Work out the finished part from the listing and answer in its coordinate system (mm). Face numbers are marked on the shaded views. A direction names the side the tool comes from. Coordinates: 2 decimals unless noted, no trailing zeros. Write each loop counter-clockwise with the first axis right and the second up, starting at its lowest first coordinate (ties: lowest second). Pieces come first, ordered by that corner, then holes. Notation, with made-up numbers: M -2,-2.75 L 16,-2.75 A8 ccw 16,3.25 Z; hole C 48,-17.75 d4. An arc over 180 degrees is marked long. Answer as CSV lines item,"result". Start each with the question number.
(1) A cutting plane is placed at C-C on z = -14. Give the vertices of the cut face in (x, y).
(2) A cutting plane is placed at A-A on x = 25. Give the vertices of the cut face in (y, z).
(3) For the marked faces 1 and 2, determine the directions among +Z, -Z, +X, -X, +Y, -Y from which every point of the face is accessible in a straight line to the end or side of a thin tool.
(4) Flat-ended cylindrical pins translate along their axes: P1, Ø1.4, axis at y = -2.37, z = -7.24, coming from the +X side; P2, Ø6, axis at x = 18.5, z = -132, coming from the +Y side; P3, Ø1.5, axis at x = 47.5, y = -3, coming from the +Z side; P4, Ø2, axis at y = -6.71, z = -3.6, coming from the -X side. Find the tip coordinate at first contact, or state that the pin passes through.
(5) A cutting plane is placed at B-B on y = 21. Give the vertices of the cut face in (x, z).
(6) Find the intervals of material crossed by L1, parallel to X at y = 9, z = -3.5; L2, parallel to X at y = -3.5, z = -79; L3, parallel to Y at x = 15, z = -22, in increasing order. Write a range as [from, to].
from build123d import *

# Parameters (mm, degrees)
BOSS_EXTRUDE1_DEPTH = 17.78
SKETCH2_R           = 10
CUT_EXTRUDE2_DEPTH  = 5.08
SKETCH8_R           = 0.75
SKETCH8_R_2         = 0.724827396
SKETCH8_R_3         = 0.742534986
CUT_EXTRUDE7_DEPTH  = 5.08
BOSS_EXTRUDE2_DEPTH = 35.56
SKETCH7_W           = 41.148
SKETCH7_H           = 20.066
CUT_EXTRUDE5_DEPTH  = 26.797
FILLET2_R           = 2.54
FILLET3_R           = 2.54
FILLET4_R           = 2.54
FILLET5_R           = 12.7


with BuildPart() as part:
    # Sketch1 → Boss-Extrude1 (new body)
    with BuildSketch(Plane(origin=(0, 0, 0), x_dir=(0, 0, -1), z_dir=(1, 0, 0))):
        with BuildLine():
            Line((32.896583501, -19.220426478), (153.708015153, -35.416630381))
            Line((153.708015153, -35.416630381), (158.7704814, 2.345538988))
            Line((158.7704814, 2.345538988), (32.896583501, 19.220426478))
            ThreePointArc((32.896583501, 19.220426478), (-38.1, 0), (32.896583501, -19.220426478))
        make_face()
    extrude(amount=BOSS_EXTRUDE1_DEPTH)

    # Sketch2 → Cut-Extrude2 (cut)
    with BuildSketch(Plane(origin=(17.78, 0, 0), x_dir=(0, 0, -1), z_dir=(1, 0, 0))):
        Circle(SKETCH2_R)
    extrude(amount=-CUT_EXTRUDE2_DEPTH, mode=Mode.SUBTRACT)

    # Sketch8 → Cut-Extrude7 (cut)
    with BuildSketch(Plane(origin=(12.7, 0, 0), x_dir=(0, 0, -1), z_dir=(1, 0, 0))):
        with Locations((-7.236662764, 2.372912145)):
            Circle(SKETCH8_R)
        with Locations((-6.97289018, -0.615469361)):
            Circle(SKETCH8_R)
        with Locations((-6.709117597, -3.603850867)):
            Circle(SKETCH8_R)
        with Locations((-2.372912145, -7.236662764)):
            Circle(SKETCH8_R)
        with Locations((0.615469361, -6.97289018)):
            Circle(SKETCH8_R)
        with Locations((3.603850867, -6.709117597)):
            Circle(SKETCH8_R)
        with Locations((7.236662764, -2.372912145)):
            Circle(SKETCH8_R)
        with Locations((6.97289018, 0.615469361)):
            Circle(SKETCH8_R)
        with Locations((6.709117597, 3.603850867)):
            Circle(SKETCH8_R_2)
        with Locations((2.372912145, 7.236662764)):
            Circle(SKETCH8_R)
        with Locations((-0.615469361, 6.97289018)):
            Circle(SKETCH8_R)
        with Locations((-3.603850867, 6.709117597)):
            Circle(SKETCH8_R_3)
    extrude(amount=-CUT_EXTRUDE7_DEPTH, mode=Mode.SUBTRACT)

    # Sketch4 → Boss-Extrude2 (add)
    with BuildSketch(Plane(origin=(17.78, 0, 0), x_dir=(0, 0, -1), z_dir=(1, 0, 0))):
        Polygon((158.7704814, 2.345538988), (153.708015153, -35.416630381), (115.945845783, -30.354164135), (121.00831203, 7.408005235), align=None)
    extrude(amount=BOSS_EXTRUDE2_DEPTH)

    # Sketch7 → Cut-Extrude5 (cut)
    with BuildSketch(Plane(origin=(0, -20.867859649, -155.658450257), x_dir=(-1, 0, 0), z_dir=(0, -0.1328731298372059, -0.9911330543207936))):
        with Locations((-26.769839531, 4.371072011)):
            Rectangle(SKETCH7_W, SKETCH7_H)
    extrude(amount=-CUT_EXTRUDE5_DEPTH, mode=Mode.SUBTRACT)

    # Fillet2
    fillet2_edges = [part.edges().sort_by_distance(p)[0] for p in [
        (17.78, -11.47307945, -118.477078906),
    ]]
    fillet(fillet2_edges, radius=FILLET2_R)

    # Fillet3
    fillet3_edges = [part.edges().sort_by_distance(p)[0] for p in [
        (53.34, 4.876772112, -139.889396715),
        (53.34, -11.47307945, -118.477078906),
        (53.34, -32.885397258, -134.826930468),
        (53.34, -16.535545697, -156.239248276),
    ]]
    fillet(fillet3_edges, radius=FILLET3_R)

    # Fillet4
    fillet4_edges = [part.edges().sort_by_distance(p)[0] for p in [
        (0, -16.535545697, -156.239248276),
    ]]
    fillet(fillet4_edges, radius=FILLET4_R)

    # Fillet5
    fillet5_edges = [part.edges().sort_by_distance(p)[0] for p in [
        (8.89, -19.220426478, -32.896583501),
        (8.89, 19.220426478, -32.896583501),
    ]]
    fillet(fillet5_edges, radius=FILLET5_R)


solid = part.part
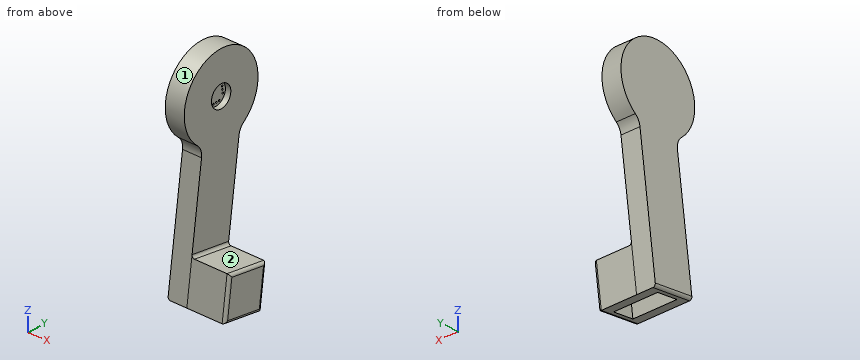
Here are the results:
1,outline,"M 0,-35.43 L 17.78,-35.43 L 17.78,35.43 L 0,35.43 Z"
2,outline,"M -35.42,-153.71 L -26.48,-154.91 L -22.92,-128.35 L -3.03,-131.01 L -6.59,-157.57 L 2.35,-158.77 L 7.41,-121.01 L -30.35,-115.95 Z"
3,face 1,"+X, -X"
3,face 2,"+Z, +X, +Y"
4,P1,"stops at x = 7.62"
4,P2,"stops at y = 6.34"
4,P3,"stops at z = -119.51"
4,P4,"stops at x = 0"
5,outline,"M 0,-32.44 L 17.78,-32.44 L 17.78,31.79 L 0,31.79 Z"
6,L1,"x = [0, 12.7]"
6,L2,"x = [0, 17.78]"
6,L3,"y = [-31.11, 31.11]"
